Model file for the job. Use its own axes, mm. A direction names the side the tool comes from. Round coordinates to 2 decimals unless told otherwise and drop trailing zeros. Order: outer loops, then holes, each group sorted by start corner. A loop starts at its lowest first (then second) coordinate and runs counter-clockwise, first axis right, second up. Notation, with made-up numbers: (82, 11) - (122, 11) arc R31 ccw to (122, 47) - close; hole circle Ø5 at (28.25, 25.5). An arc over 180 degrees is marked (long way). Use one line per item in the form item = value.
from build123d import *

# Parameters (mm, degrees)
SKETCH1_R           = 2.55
BOSS_EXTRUDE1_DEPTH = 3
CHAMFER1_SIZE       = 0.876505316
CHAMFER1_SIZE_2     = 0.8


with BuildPart() as part:
    # Sketch1 → Boss-Extrude1 (new body)
    with BuildSketch(Plane(origin=(0, 0, 0), x_dir=(1, 0, 0), z_dir=(0, 1, 0))):
        with BuildLine():
            Line((25.4, -66.8), (-25.4, -66.8))
            ThreePointArc((-25.4, -66.8), (-28.652691193, -65.452691193), (-30, -62.2))
            Line((-30, -62.2), (-30, 25.1))
            ThreePointArc((-30, 25.1), (-28.652691193, 28.352691193), (-25.4, 29.7))
            Line((-25.4, 29.7), (25.4, 29.7))
            ThreePointArc((25.4, 29.7), (28.652691193, 28.352691193), (30, 25.1))
            Line((30, 25.1), (30, -62.2))
            ThreePointArc((30, -62.2), (28.652691193, -65.452691193), (25.4, -66.8))
        make_face()
        with Locations(Location((-23.57, 23.57, 0), (0, 0, 270))):
            Circle(SKETCH1_R, mode=Mode.SUBTRACT)
        with Locations(Location((23.57, 23.57, 0), (0, 0, 90))):
            Circle(SKETCH1_R, mode=Mode.SUBTRACT)
        with Locations(Location((23.57, -23.57, 0), (0, 0, 270))):
            Circle(SKETCH1_R, mode=Mode.SUBTRACT)
        with Locations(Location((-23.57, -23.57, 0), (0, 0, 90))):
            Circle(SKETCH1_R, mode=Mode.SUBTRACT)
        with BuildLine():
            Line((17.45, -58.75), (17.45, -37.25))
            ThreePointArc((17.45, -37.25), (20, -34.7), (22.55, -37.25))
            Line((22.55, -37.25), (22.55, -58.75))
            ThreePointArc((22.55, -58.75), (20, -61.3), (17.45, -58.75))
        make_face(mode=Mode.SUBTRACT)
        with BuildLine():
            Line((7.45, -58.75), (7.45, -37.25))
            ThreePointArc((7.45, -37.25), (10, -34.7), (12.55, -37.25))
            Line((12.55, -37.25), (12.55, -58.75))
            ThreePointArc((12.55, -58.75), (10, -61.3), (7.45, -58.75))
        make_face(mode=Mode.SUBTRACT)
        with BuildLine():
            Line((-2.55, -58.75), (-2.55, -37.25))
            ThreePointArc((-2.55, -37.25), (0, -34.7), (2.55, -37.25))
            Line((2.55, -37.25), (2.55, -58.75))
            ThreePointArc((2.55, -58.75), (0, -61.3), (-2.55, -58.75))
        make_face(mode=Mode.SUBTRACT)
        with BuildLine():
            Line((-12.55, -58.75), (-12.55, -37.25))
            ThreePointArc((-12.55, -37.25), (-10, -34.7), (-7.45, -37.25))
            Line((-7.45, -37.25), (-7.45, -58.75))
            ThreePointArc((-7.45, -58.75), (-10, -61.3), (-12.55, -58.75))
        make_face(mode=Mode.SUBTRACT)
        with BuildLine():
            Line((-22.55, -58.75), (-22.55, -37.25))
            ThreePointArc((-22.55, -37.25), (-20, -34.7), (-17.45, -37.25))
            Line((-17.45, -37.25), (-17.45, -58.75))
            ThreePointArc((-17.45, -58.75), (-20, -61.3), (-22.55, -58.75))
        make_face(mode=Mode.SUBTRACT)
        with BuildLine():
            Line((14.36862915, 16.63137085), (12.326897984, 14.589639684))
            ThreePointArc((12.326897984, 14.589639684), (0, 19.1), (-12.326897984, 14.589639684))
            Line((-12.326897984, 14.589639684), (-14.36862915, 16.63137085))
            ThreePointArc((-14.36862915, 16.63137085), (-16.63137085, 16.63137085), (-16.63137085, 14.36862915))
            Line((-16.63137085, 14.36862915), (-14.589639684, 12.326897984))
            ThreePointArc((-14.589639684, 12.326897984), (-19.1, 0), (-14.589639684, -12.326897984))
            Line((-14.589639684, -12.326897984), (-16.63137085, -14.36862915))
            ThreePointArc((-16.63137085, -14.36862915), (-16.63137085, -16.63137085), (-14.36862915, -16.63137085))
            Line((-14.36862915, -16.63137085), (-12.326897984, -14.589639684))
            ThreePointArc((-12.326897984, -14.589639684), (0, -19.1), (12.326897984, -14.589639684))
            Line((12.326897984, -14.589639684), (14.36862915, -16.63137085))
            ThreePointArc((14.36862915, -16.63137085), (16.63137085, -16.63137085), (16.63137085, -14.36862915))
            Line((16.63137085, -14.36862915), (14.589639684, -12.326897984))
            ThreePointArc((14.589639684, -12.326897984), (19.1, 0), (14.589639684, 12.326897984))
            Line((14.589639684, 12.326897984), (16.63137085, 14.36862915))
            ThreePointArc((16.63137085, 14.36862915), (16.63137085, 16.63137085), (14.36862915, 16.63137085))
        make_face(mode=Mode.SUBTRACT)
    extrude(amount=BOSS_EXTRUDE1_DEPTH)

    # Chamfer1
    # the kernel refuses this chamfer: 0.876505316, 0.8 mm, written as the material it takes off along each edge
    with BuildSketch(Plane(origin=(-14.589639684, -2.258924043, -12.326897984), x_dir=(-0.7071067811865476, 0, -0.7071067811865476), z_dir=(0, 1, 0)), Plane(origin=(-12.326897984, -2.258924043, 14.589639684), x_dir=(-0.7071067811865435, 0, 0.7071067811865516), z_dir=(0, 1, 0)), Plane(origin=(14.589639684, -2.258924043, 12.326897984), x_dir=(0.7071067811865475, 0, 0.7071067811865475), z_dir=(0, 1, 0)), Plane(origin=(12.326897984, -2.258924043, -14.589639684), x_dir=(0.7071067811865465, 0, -0.7071067811865486), z_dir=(0, 1, 0))) as chamfer1_piece_1:
        with BuildLine():
            Line((CHAMFER1_SIZE, 0), (-0.085923492, 0.81316345))
            ThreePointArc((-0.085923492, 0.81316345), (-0.039945159, 0.419640102), (0, 0))
            Line((0, 0), (CHAMFER1_SIZE, 0))
        make_face()
    extrude(amount=7.517848085, mode=Mode.SUBTRACT)
    with BuildSketch(Plane(origin=(-14.589639684, -2.323826689, 12.326897984), x_dir=(-0.6271715557767805, 0, -0.7788811460194248), z_dir=(0, 1, 0)), Plane(origin=(12.326897984, -2.323826689, 14.589639684), x_dir=(-0.7788811460194289, 0, 0.6271715557767755), z_dir=(0, 1, 0)), Plane(origin=(14.589639684, -2.323826689, -12.326897984), x_dir=(0.6271715557767805, 0, 0.7788811460194248), z_dir=(0, 1, 0)), Plane(origin=(-12.326897984, -2.323826689, -14.589639684), x_dir=(0.7788811460194278, 0, -0.6271715557767769), z_dir=(0, 1, 0))) as chamfer1_piece_2:
        with BuildLine():
            Line((0.90196282, 0), (-CHAMFER1_SIZE_2 * 0.107274880032, CHAMFER1_SIZE_2 * 0.994229400146))
            Line((-CHAMFER1_SIZE_2 * 0.107274880032, CHAMFER1_SIZE_2 * 0.994229400146), (0, 0))
            ThreePointArc((0, 0), (0.464646952, 0.005320048), (0.90196282, 0))
        make_face()
    extrude(amount=7.647653377, mode=Mode.SUBTRACT)


solid = part.part
(1) Slice it at D-D on x = -6.5. Give the cut face in (y, z).
Report:
outline = (0, -29.7) - (3, -29.7) - (3, -17.96) - (0, -17.96) - close; (0, 17.96) - (3, 17.96) - (3, 66.8) - (0, 66.8) - close
(2) Slice it at C-C on z = 54.5. Give the cut face in (x, y).
Report:
outline = (-30, 0) - (-22.55, 0) - (-22.55, 3) - (-30, 3) - close; (-17.45, 0) - (-12.55, 0) - (-12.55, 3) - (-17.45, 3) - close; (-7.45, 0) - (-2.55, 0) - (-2.55, 3) - (-7.45, 3) - close; (2.55, 0) - (7.45, 0) - (7.45, 3) - (2.55, 3) - close; (12.55, 0) - (17.45, 0) - (17.45, 3) - (12.55, 3) - close; (22.55, 0) - (30, 0) - (30, 3) - (22.55, 3) - close
(3) Probe probe 1 along X at (y, z) = (1, 23.57); probe 2 along X at (y, z) = (2.2, 44); probe 3 along Z at (x, y) = (-25.5, 2.4). List the from-to ranges inside material, lowest first. Write a range as [from, to].
Report:
probe_1 = [-30, -26.12], [-21.02, 21.02], [26.12, 30]
probe_2 = [-30, -22.55], [-17.45, -12.55], [-7.45, -2.55], [2.55, 7.45], [12.55, 17.45], [22.55, 30]
probe_3 = [-29.7, -25.24], [-21.9, 21.9], [25.24, 66.8]
(4) Pin check, flat tip, straight feed: pin 1 (4.5 mm diameter, centred on x = 23.57, z = 23.57, fed in from -Y). Stop position of the tip, or through.
Report:
pin_1 = through
(5) Slice it at A-A on x = 23.57. Give the cut face in (y, z), then the cut area to 3 significant figures.
Report:
outline = (0, -29.7) - (3, -29.7) - (3, -26.12) - (0, -26.12) - close; (0, -21.02) - (3, -21.02) - (3, 21.02) - (0, 21.02) - close; (0, 26.12) - (3, 26.12) - (3, 66.8) - (0, 66.8) - close
area = 259 mm2
(6) Slice it at B-B on z = -23.57. Give the cut face in (x, y).
Report:
outline = (-30, 0) - (-26.12, 0) - (-26.12, 3) - (-30, 3) - close; (-21.02, 0) - (21.02, 0) - (21.02, 3) - (-21.02, 3) - close; (26.12, 0) - (30, 0) - (30, 3) - (26.12, 3) - close
(7) Tool access for faces 5 (the face through (28.688, 1.479, 65.417)), 6 (the face through (-9.9, 1.5, 61.3)): list every direction of +Z, -Z, +X, -X, +Y, -Y with a clear straight run to the whole face (end or side of a thin tool).
Report:
face_5 = +Z, +X, +Y, -Y
face_6 = +Y, -Y
(8) Pull direction Z, two halves, no side cores. Call faces 1 (the face through (-19.9, 1.5, 61.3)), 2 (the face through (7, 3, 18)), 3 (the face through (-28.617, 1.479, 65.488)), 4 (the face through (0, 1, -29.7)): released by +Z, released by -Z, zero draft, split by the parting line, or undercut.
Report:
face_1 = undercut
face_2 = zero draft
face_3 = released by +Z
face_4 = released by -Z
